from build123d import *

# Parameters (mm, degrees)
SKETCH1_W                      = 240.6
SKETCH1_H                      = 180.2
BOSS_EXTRUDE1_DEPTH            = 8
SKETCH2_W                      = 160.6
SKETCH2_H                      = 100.2
CUT_EXTRUDE1_DEPTH             = 200.503872501
CUT_EXTRUDE2_DEPTH             = 7
CUT_EXTRUDE3_DEPTH             = 7
CUT_EXTRUDE4_DEPTH             = 7
CUT_EXTRUDE5_DEPTH             = 7
F_6_5_6_5_DIAMETER_HOLE1_D     = 6.5
F_6_5_6_5_DIAMETER_HOLE1_DEPTH = 8
SKETCH9_R                      = 9.267416037
SKETCH9_R_2                    = 9.269178346
SKETCH9_R_3                    = 9.266671768
CUT_EXTRUDE7_DEPTH             = 4
SKETCH10_R                     = 1.5
CUT_EXTRUDE8_DEPTH             = 0.5


with BuildPart() as part:
    # Sketch1 → Boss-Extrude1 (new body)
    with BuildSketch(Plane(origin=(0, 0, 0), x_dir=(-1, 0, 0), z_dir=(0, 0, -1))):
        with Locations((-50.702318109, 12.34999924)):
            Rectangle(SKETCH1_W, SKETCH1_H)
    extrude(amount=-BOSS_EXTRUDE1_DEPTH)

    # Sketch2 → Cut-Extrude1 (cut, through all)
    with BuildSketch(Plane.XY.offset(8)):
        with Locations((50.702318109, 12.34999924)):
            Rectangle(SKETCH2_W, SKETCH2_H)
    extrude(amount=-CUT_EXTRUDE1_DEPTH, mode=Mode.SUBTRACT)

    # Sketch3 → Cut-Extrude2 (cut)
    with BuildSketch(Plane(origin=(0, 0, 0), x_dir=(-1, 0, 0), z_dir=(0, 0, -1))):
        Polygon((-117.686768689, -48.483328992), (-127.060792146, -58.198146757), (-117.921667286, -67.016672528), (-108.547643828, -57.301854763), align=None)
    extrude(amount=-CUT_EXTRUDE2_DEPTH, mode=Mode.SUBTRACT)

    # Sketch4 → Cut-Extrude3 (cut)
    with BuildSketch(Plane(origin=(0, 0, 0), x_dir=(-1, 0, 0), z_dir=(0, 0, -1))):
        Polygon((6.939207854, -58.198146757), (16.078332714, -67.016672528), (25.452356172, -57.301854763), (16.313231311, -48.483328992), align=None)
    extrude(amount=-CUT_EXTRUDE3_DEPTH, mode=Mode.SUBTRACT)

    # Sketch5 → Cut-Extrude4 (cut)
    with BuildSketch(Plane(origin=(0, 0, 0), x_dir=(-1, 0, 0), z_dir=(0, 0, -1))):
        Polygon((-37.727458813, -58.198146757), (-28.588333952, -67.016672528), (-19.214310494, -57.301854763), (-28.353435355, -48.483328992), align=None)
    extrude(amount=-CUT_EXTRUDE4_DEPTH, mode=Mode.SUBTRACT)

    # Sketch6 → Cut-Extrude5 (cut)
    with BuildSketch(Plane(origin=(0, 0, 0), x_dir=(-1, 0, 0), z_dir=(0, 0, -1))):
        Polygon((-82.39412548, -58.198146757), (-73.255000619, -67.016672528), (-63.880977161, -57.301854763), (-73.020102022, -48.483328992), align=None)
    extrude(amount=-CUT_EXTRUDE5_DEPTH, mode=Mode.SUBTRACT)

    # Ø6.5 (6.5) Diameter Hole1
    with Locations(Plane.XY.offset(8)):
        with Locations((117.804217987, -57.75000076), (-16.097681891, -57.75000076), (28.568984776, -57.75000076), (73.235651442, -57.75000076)):
            Hole(F_6_5_6_5_DIAMETER_HOLE1_D / 2, depth=F_6_5_6_5_DIAMETER_HOLE1_DEPTH)

    # Sketch9 → Cut-Extrude7 (cut)
    with BuildSketch(Plane(origin=(0, 0, 0), x_dir=(-1, 0, 0), z_dir=(0, 0, -1))):
        with Locations((-117.804217987, -57.75000076)):
            Circle(SKETCH9_R)
        with Locations((-73.235651442, -57.75000076)):
            Circle(SKETCH9_R_2)
        with Locations((-28.568984776, -57.75000076)):
            Circle(SKETCH9_R_2)
        with Locations((16.097681891, -57.75000076)):
            Circle(SKETCH9_R_3)
    extrude(amount=-CUT_EXTRUDE7_DEPTH, mode=Mode.SUBTRACT)

    # Sketch10 → Cut-Extrude8 (cut)
    with BuildSketch(Plane(origin=(0, 0, 0), x_dir=(-1, 0, 0), z_dir=(0, 0, -1))):
        with Locations((-127.002318109, 69.24999924)):
            Circle(SKETCH10_R)
        with Locations((29.997681891, 69.24999924)):
            Circle(SKETCH10_R)
        with Locations((29.997681891, -45.75000076)):
            Circle(SKETCH10_R)
        with Locations((-127.002318109, -45.75000076)):
            Circle(SKETCH10_R)
    extrude(amount=-CUT_EXTRUDE8_DEPTH, mode=Mode.SUBTRACT)


solid = part.part
Could you check a few things on this model? Use its own coordinates, in mm. A direction names the side the tool comes from. Give positions to 0.01 mm unless a question says otherwise; leave off trailing zeros. Write each loop counter-clockwise with the first axis right and the second up, starting at its lowest first coordinate (ties: lowest second). Pieces come first, ordered by that corner, then holes. Notation, with made-up numbers: (-4.5, -24) -> (3.5, -24) arc R16 cw to (3.5, -17) -> close; hole circle Ø1 at (14.5, -0.5). An arc over 180 degrees is marked (long way). Write each question's results on one line, items separated by ' | '. Start each with the question number.
Q1. We'd pull the mould along Y, two halves only. Please class faces 1 (the face through (52, 74, 8)), 2 (the face through (52, 102.45, 4)), 3 (the face through (-20.7, -62.227, 5.007)), 4 (the face through (68.39, -52.95, 5.01)): +Y half, -Y half, draft (parallel to the pull), parting line (faces both ways), or undercut.
Q2. Which directions (+Z, -Z, +X, -X, +Y, -Y) give clear straight access to the entire face, cutting with the end or side of a thin tool? Please do faces 5 (the face through (-22.69, -64.26, 1.97)), 6 (the face through (50, -37.75, 4)).
Q3. Suppose I cut it at B-B, the plane y = 24.5. List the corners of the cut face in (x, z) for me.
Q4. I'm going to push flat-ended pins straight in: pin 1 Ø7.5 at (x, y) = (-19, -60) entering from -Z; pin 2 Ø4.5 at (x, y) = (-12.5, -60) entering from -Z. Where does each tip first touch, or does it pass through?
Q5. I need wall thicknesses on probe 1 along X at (y, z) = (69.25, 0.4); probe 2 along X at (y, z) = (-57.75, 7.5); probe 3 along Y at (x, z) = (-1, 5). Which ranges of each line are inside material? Lowest first, please.
Q6. Suppose I cut it at A-A, the plane x = 8.5. List the corners of the cut face in (y, z) for me, and give its area (3 significant figures).
Outcome:
1) face 1: draft | face 2: +Y half | face 3: undercut | face 4: undercut
2) face 5: -Z | face 6: +Z, -Z
3) outline: (-69.6, 0) -> (-29.6, 0) -> (-29.6, 8) -> (-69.6, 8) -> close; (131, 0) -> (171, 0) -> (171, 8) -> (131, 8) -> close
4) pin 1: z = 4 | pin 2: z = 7
5) probe 1: -69.6 to -31.5, -28.5 to 125.5, 128.5 to 171 | probe 2: -69.6 to -19.35, -12.85 to 25.32, 31.82 to 69.99, 76.49 to 114.55, 121.05 to 171 | probe 3: -77.75 to -37.75, 62.45 to 102.45
6) outline: (-77.75, 0) -> (-37.75, 0) -> (-37.75, 8) -> (-77.75, 8) -> close; (62.45, 0) -> (102.45, 0) -> (102.45, 8) -> (62.45, 8) -> close | area: 640 mm2
